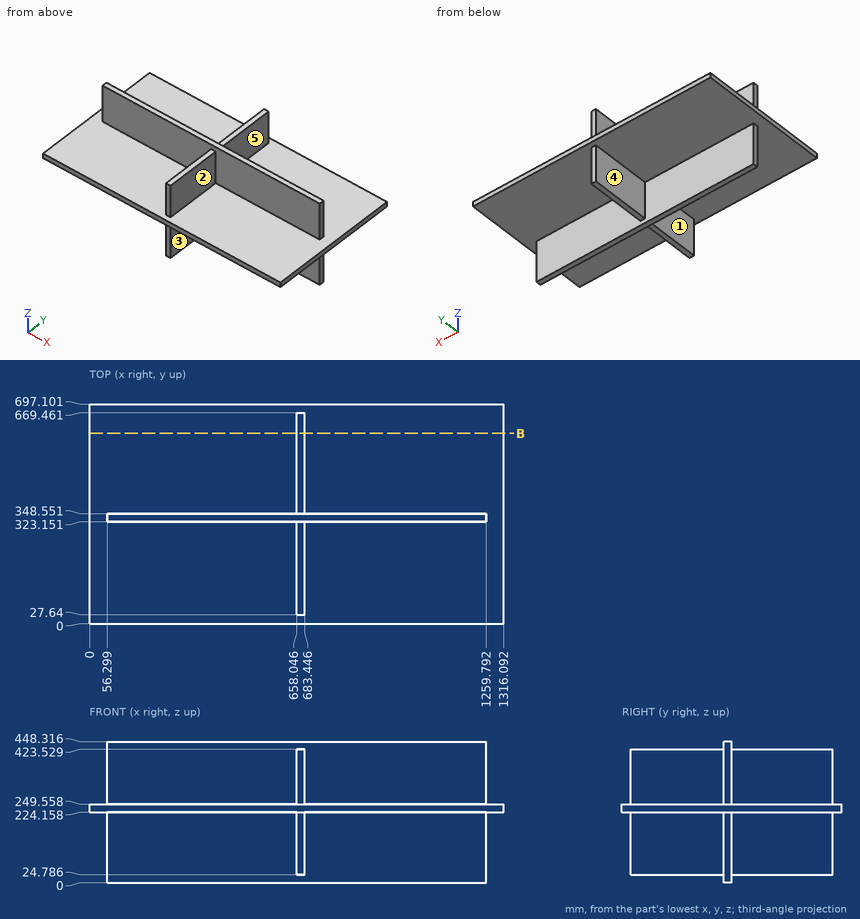
Geometry: see drawing. Coordinates: mm, zero at the bounding-box minimum. A direction names the side the tool comes from. Give positions to 0.01 mm unless a question says otherwise; leave off trailing zeros. Order: outer loops, then holes, each group sorted by start corner. A loop starts at its lowest first (then second) coordinate and runs counter-clockwise, first axis right, second up. Notation, with made-up numbers: (81.25, 71.5) - (86.25, 71.5) arc R24 ccw to (86.25, 88.5) - close; hole circle Ø1 at (41.5, 69.25). An arc over 180 degrees is marked (long way). Write each question's results on one line, items separated by ' | '.
Item 1: Section B-B (y = 604). Return loops of the section in (x, z) (1 decimal), and give its area (3 significant figures).
A:
outline: (0, 224.2) - (658, 224.2) - (658, 24.8) - (683.4, 24.8) - (683.4, 224.2) - (1316.1, 224.2) - (1316.1, 249.6) - (683.4, 249.6) - (683.4, 423.5) - (658, 423.5) - (658, 249.6) - (0, 249.6) - close | area: 42,900 mm^2
Item 2: Material intervals for line 1 along Y through (x, z) = (735, 59); line 2 along X through (y, z) = (175, 301) (1 decimal); line 3 along Z through (x, y) = (109, 227.5), sorted ascending.
A:
line 1: y = 323.15 to 348.55 | line 2: x = 658 to 683.4 | line 3: z = 224.16 to 249.56
Item 3: Contact query for flat-ended pins moving along their axis: pin 1 Ø20.5 at (x, y) = (665, 564) entering from +Z; pin 2 Ø12.5 at (x, z) = (667, 149.5) entering from -Y; pin 3 Ø8 at (x, z) = (555, 216.5) entering from -Y. Output: stop coordinate, or through.
A:
pin 1: stops at z = 423.53 | pin 2: stops at y = 27.64 | pin 3: stops at y = 323.15
Item 4: Access query for the marked faces 1, 2, 3, 4 and 5. Directions: +Z, -Z, +X, -X, +Y, -Y. A direction counts if a zero-diameter tool reaches every point of the face in a straight line with its end or side. Return the directions, or none.
A:
face 1: -Z, -X, -Y | face 2: +Z, +X, -Y | face 3: -Z, +X, -Y | face 4: -Z, -X, +Y | face 5: +Z, +X, +Y
